```python
from build123d import *

# Parameters (mm, degrees)
F0_W     = 10
F0_H     = 12
F1_DEPTH = 26
F2_R     = 1.5
F3_DEPTH = 9.27
F4_R     = 0.8
F5_DEPTH = 3


with BuildPart() as f1:
    # F0 (on Top) → F1 (new body)
    with BuildSketch(Plane.XY):
        Rectangle(F0_W, F0_H)
    extrude(amount=F1_DEPTH)

    # F2 (on face) → F3 (join)
    with BuildSketch(Plane.XY.offset(26)):
        Circle(F2_R)
    extrude(amount=F3_DEPTH)

    # F4 (on face) → F5 (cut)
    with BuildSketch(Plane.XY.offset(26)):
        with Locations((0, 4.5)):
            Circle(F4_R)
        with Locations((0, -4.5)):
            Circle(F4_R)
    extrude(amount=-F5_DEPTH, mode=Mode.SUBTRACT)


solid = f1.part
```
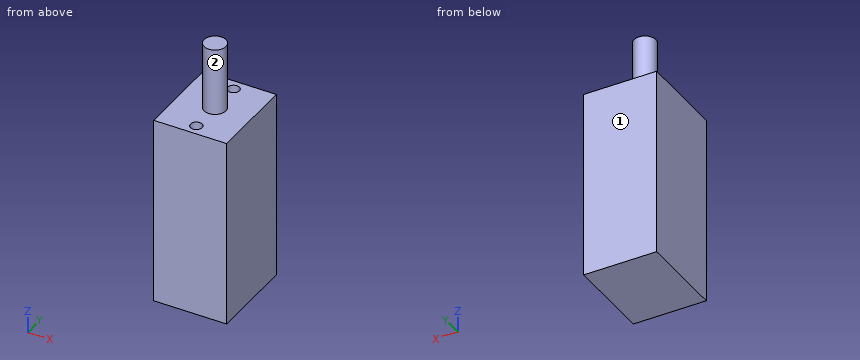
Work out the finished part from the listing and answer in its coordinate system (mm). Face numbers are marked on the shaded views. A direction names the side the tool comes from. Give positions to 0.01 mm unless a question says otherwise; leave off trailing zeros. Loops run counter-clockwise (first coordinate to the right, second up) from the corner with the lowest first, then second, coordinate; pieces in that order, holes last. Notation, with made-up numbers: (-39, -31.5) -> (-6, -31.5) arc R23 cw to (-6, -3.5) -> close; hole circle Ø1 at (73, -24.5). An arc over 180 degrees is marked (long way). Write item = value, one per line. Start each with the question number.
(1) Given pin 1 Ø1.8 at (x, y) = (0, 4.5) entering from +Z, flat-ended and moving along its own axis, determine where the tip first touches the part or whether it passes through.
(2) Find section C-C on y = 0. Give the vertices of the cut face in (x, z).
(3) Find section D-D on x = 4. Give the vertices of the cut face in (y, z).
(4) Which of the six approach directions +Z, -Z, +X, -X, +Y, -Y give full straight-line access (tool end or side, diameter ignored) to the marked faces 1 and 2?
(5) Find the intervals of material crossed by probe 1 along Y at (x, z) = (0, 23.9); probe 2 along Z at (x, y) = (-3.5, -1.25); probe 3 along Z at (x, y) = (-0.5, -4), in increasing order. Write a range as from..to.
(6) Find section B-B on x = 0. Give the vertices of the cut face in (y, z).
(7) Find section A-A on y = 4.5. Give the vertices of the cut face in (x, z), and give its area (3 significant figures).
From the geometry:
q1.pin_1 = 26
q2.outline = (-5, 0) -> (5, 0) -> (5, 26) -> (1.5, 26) -> (1.5, 35.27) -> (-1.5, 35.27) -> (-1.5, 26) -> (-5, 26) -> close
q3.outline = (-6, 0) -> (6, 0) -> (6, 26) -> (-6, 26) -> close
q4.face_1 = +Z, -Z, +X, -X, +Y
q4.face_2 = +Z
q5.probe_1 = -6..-5.3, -3.7..3.7, 5.3..6
q5.probe_2 = 0..26
q5.probe_3 = 0..23
q6.outline = (-6, 0) -> (6, 0) -> (6, 26) -> (5.3, 26) -> (5.3, 23) -> (3.7, 23) -> (3.7, 26) -> (1.5, 26) -> (1.5, 35.27) -> (-1.5, 35.27) -> (-1.5, 26) -> (-3.7, 26) -> (-3.7, 23) -> (-5.3, 23) -> (-5.3, 26) -> (-6, 26) -> close
q7.outline = (-5, 0) -> (5, 0) -> (5, 26) -> (0.8, 26) -> (0.8, 23) -> (-0.8, 23) -> (-0.8, 26) -> (-5, 26) -> close
q7.area = 255 mm^2
